Read the model definition and answer for the solid it produces. Units are mm, in the model's axes. A direction names the side the tool comes from. Coordinates: 2 decimals unless noted, no trailing zeros. Loops run counter-clockwise (first coordinate to the right, second up) from the corner with the lowest first, then second, coordinate; pieces in that order, holes last. Notation, with made-up numbers: (72, -35) - (82, -35) arc R21 ccw to (82, -16) - close; hole circle Ø11 at (-8.5, -39.75). An arc over 180 degrees is marked (long way). Use one line per item in the form item = value. Start each with the question number.
1) Consider line 1 (X direction, y = 19, z = 3.5); line 2 (X direction, y = -21.5, z = 3.25); line 3 (Y direction, x = -78, z = 8.25). Determine where each line is inside the solid, lowest interval first.
2) The mould has two halves that part along X. Classify faces 3 (the face through (84, 23, 5)), 4 (the face through (-85, -3, 5)), 5 (the face through (-75.6, 19.53, 4.93)): released by +X, released by -X, zero draft, split by the parting line, or undercut.
3) A cutting plane is placed at A-A (y = -17.5). Give the vertices of the cut face in (x, z), and give its area (3 significant figures).
4) Each of these flat-tipped pins is pushed along its axis until it touches: P1, Ø10, axis at x = -67, y = 17.5, coming from the -Z side; P2, Ø4.5, axis at x = 78, y = 19, coming from the -Z side. Where does it stop, or does it pass through?
5) Which of the six approach directions +Z, -Z, +X, -X, +Y, -Y give full straight-line access (tool end or side, diameter ignored) to faces 1 (the face through (80.4, -17.4, 5.53)), 2 (the face through (85, -2, 5))?
Autodesk Inventor part; units mm, degrees
ref_plane "YZ Plane" through (0, 0, 0) normal (1, 0, 0) x (0, 1, 0)
ref_plane "XZ Plane" through (0, 0, 0) normal (0, 1, 0) x (-1, 0, 0)
ref_plane "XY Plane" through (0, 0, 0) normal (0, 0, 1) x (1, 0, 0)
sketch "Sketch1" plane through (0, 0, 0) normal (0, 0, 1) x (1, 0, 0)
  line L0 (85, -25) -> (-85, -25)
  line L1 (-85, -25) -> (-85, 25)
  line L2 (-85, 25) -> (85, 25)
  line L3 (85, 25) -> (85, -25)
  line L4 (85, -25) -> (-85, 25) construction
  line L5 (-85, -25) -> (85, 25) construction
  point P0 (0, 0)
  dimension "d0" = 170
  dimension "d1" = 50
extrude "Extrusion1" add sketch "Sketch1" along normal blind 10
sketch "Sketch2" plane through (0, 0, 10) normal (0, 0, 1) x (1, 0, 0)
  line L0 (85, 25) -> (-85, 25) construction
  line L1 (0, 25) -> (0, -25) construction
  line L2 (-85, -25) -> (85, -25) construction
  line L3 (-85, 25) -> (-85, -25)
  line L4 (85, -25) -> (85, 25)
  point P0 (0, 0)
  point P1 (-78, 19)
  point P2 (78, 19)
  dimension "d4" = 7
  dimension "d5" = 6
hole "Hole1" at (-78, 19, 10) at (78, 19, 10) direction (0, 0, -1) diameter 4.917 end through all
sketch "Sketch3" plane through (-85, -25, 0) normal (0, -1, 0) x (1, 0, 0)
  line L0 (0, 0) -> (0, 10)
  line L1 (0, 10) -> (170, 10)
  line L2 (85, 0) -> (85, 10) construction
  point P0 (7, 5)
  point P1 (0, 5)
  point P2 (163, 5)
  dimension "d24" = 5
  dimension "d25" = 7
hole "Hole2" at (-78, -25, 5) at (78, -25, 5) direction (0, 1, 0) diameter 4.917 depth 15 tip angle 118
fillet "Fillet1" radius 5 2 edges at (-85, 25, 5) (85, 25, 5)
properties part number "Support_driver" material "Stainless Steel"
Found:
q1.line_1 = -85 to -80.46, -75.54 to 75.54, 80.46 to 85
q1.line_2 = -85 to -79.73, -76.27 to 76.27, 79.73 to 85
q1.line_3 = -25 to 16.54, 21.46 to 25
q2.face_3 = released by +X
q2.face_4 = released by -X
q2.face_5 = undercut
q3.outline = (-85, 0) - (85, 0) - (85, 10) - (-85, 10) - close; hole circle Ø4.92 at (-78, 5); hole circle Ø4.92 at (78, 5)
q3.area = 1,660 mm^2
q4.P1 = 0
q4.P2 = through
q5.face_1 = -Y
q5.face_2 = +Z, -Z, +X, +Y, -Y
